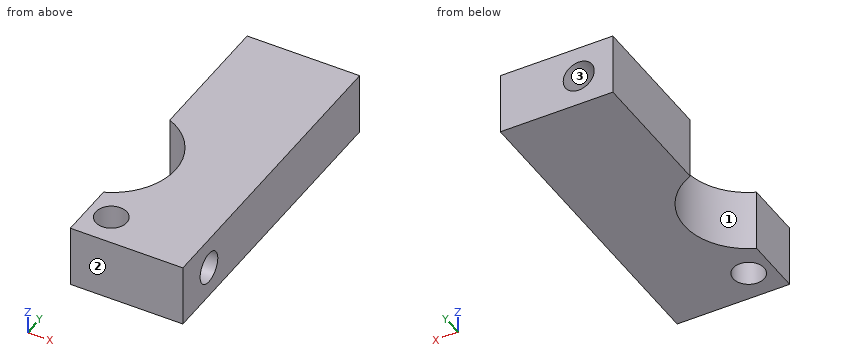
Autodesk Inventor part; units mm, degrees
ref_plane "YZ Plane" through (0, 0, 0) normal (1, 0, 0) x (0, 1, 0)
ref_plane "XZ Plane" through (0, 0, 0) normal (0, 1, 0) x (-1, 0, 0)
ref_plane "XY Plane" through (0, 0, 0) normal (0, 0, 1) x (1, 0, 0)
sketch "Эскиз1" plane through (0, 0, 0) normal (0, 0, 1) x (1, 0, 0)
  line L0 (0, 0) -> (-14.5, 0)
  line L1 (-14.5, 0) -> (-14.5, 40)
  line L2 (-14.5, 40) -> (0, 40)
  line L3 (0, 40) -> (0, 0)
  circle A0 centre (-11.5, 4) radius 2
  arc A1 (-14.5, 7.5) -> (-14.5, 22.5) centre (-17.6022, 15) ccw
  dimension "d0" = 14.5
  dimension "d1" = 40
  dimension "d2" = 4
  dimension "d4" = 4
  dimension "d5" = 11.5
  dimension "d6" = 15
  dimension "d7" = 15
extrude "Выдавливание1" add sketch "Эскиз1" along normal mid plane 8 contours L0 L1 A1 L2 L3
sketch "Эскиз2" plane through (0, 0, 4) normal (1, 0, 0) x (0, 0, -1)
  circle A0 centre (4, 5.9) radius 2
  line L0 (4, 0) -> (4, 4.8588) construction
  line L1 (8, 0) -> (0, 0)
  dimension "d10" = 4
  dimension "d16" = 5.9
extrude "Выдавливание2" cut sketch "Эскиз2" against normal blind 5
sketch "Эскиз3" plane through (-14.5, 40, 4) normal (0, 1, 0) x (1, 0, 0)
  circle A0 centre (4.4, 4) radius 2
  line L0 (14.5, 4) -> (4.4, 4) construction
  line L1 (14.5, 8) -> (14.5, 0)
  dimension "d13" = 4
  dimension "d17" = 10.1
extrude "Выдавливание3" cut sketch "Эскиз3" against normal blind 5
properties part number "держатель шкива"
Part model, mm, in its own coordinate system. Face numbers are marked on the shaded views. Give positions to 0.01 mm unless a question says otherwise; leave off trailing zeros. Order: outer loops, then holes, each group sorted by start corner. A loop starts at its lowest first (then second) coordinate and runs counter-clockwise, first axis right, second up. Notation, with made-up numbers: (61, 60) - (91, 60) arc R21 cw to (91, 87) - close; hole circle Ø6 at (43, 81.25). An arc over 180 degrees is marked (long way). Use a Markdown table: item, result.
1) Flat gauge pins, fed straight in: P1, Ø2, axis at y = 5, z = 0, coming from the +X side; P2, Ø3.5, axis at x = -11.5, y = 4, coming from the -Z side. Where does each tip first touch, or does it go through?
Checked values:
| item | result |
|---|---|
| P1 | x = -5 |
| P2 | through |
2) Saw through at D-D on z = 0. List the corners of the cut face in (x, y).
Checked values:
| item | result |
|---|---|
| outline | (-14.5, 0) - (0, 0) - (0, 3.9) - (-5, 3.9) - (-5, 7.9) - (0, 7.9) - (0, 40) - (-8.1, 40) - (-8.1, 35) - (-12.1, 35) - (-12.1, 40) - (-14.5, 40) - (-14.5, 22.5) arc R8.12 cw to (-14.5, 7.5) - close; hole circle Ø4 at (-11.5, 4) |
3) Two-plate mould, pull along Y, no slides. Class the marked faces 1, 2 and 3: +Y half, -Y half, draft (parallel to the pull), parting line (faces both ways), or undercut.
Checked values:
| item | result |
|---|---|
| face 1 | undercut |
| face 2 | -Y half |
| face 3 | draft |
4) Saw through at C-C on x = -2. List the corners of the cut face in (y, z).
Checked values:
| item | result |
|---|---|
| outline | (0, -4) - (40, -4) - (40, 4) - (0, 4) - close; hole circle Ø4 at (5.9, 0) |
5) Saw through at B-B on x = -11.5. List the corners of the cut face in (y, z).
Checked values:
| item | result |
|---|---|
| outline | (0, -4) - (2, -4) - (2, 4) - (0, 4) - close; (6, -4) - (9.65, -4) - (9.65, 4) - (6, 4) - close; (20.35, -4) - (40, -4) - (40, -1.43) - (35, -1.43) - (35, 1.43) - (40, 1.43) - (40, 4) - (20.35, 4) - close |
6) Probe L1, parallel to X at y = 38.35, z = 0; L2, parallel to Y at x = -2, z = 0; L3, parallel to Z at x = -10.1, y = 36.1. List the from-to ranges inside material, lowest first. Write a range as from..to.
Checked values:
| item | result |
|---|---|
| L1 | -14.5..-12.1, -8.1..0 |
| L2 | 0..3.9, 7.9..40 |
| L3 | -4..-2, 2..4 |
7) Saw through at A-A on z = 2.5. List the corners of the cut face in (x, y).
Checked values:
| item | result |
|---|---|
| outline | (-14.5, 0) - (0, 0) - (0, 40) - (-14.5, 40) - (-14.5, 22.5) arc R8.12 cw to (-14.5, 7.5) - close; hole circle Ø4 at (-11.5, 4) |
